```python
from build123d import *

# Parameters (mm, degrees)
F1_DEPTH = 10
F3_DEPTH = 4
F4_DEPTH = 4


with BuildPart() as f1:
    # F0 (on Top) → F1 (new body)
    with BuildSketch(Plane.XY):
        with BuildLine():
            Line((115, 150), (115, 0))
            Line((115, 0), (125, 0))
            Line((125, 0), (125, 150))
            ThreePointArc((125, 150), (0, 185), (-125, 150))
            Line((-125, 150), (-125, 0))
            Line((-125, 0), (-115, 0))
            Line((-115, 0), (-115, 150))
            Line((-115, 150), (-104.454365, 150))
            ThreePointArc((-104.454365, 150), (0, 175), (104.454365, 150))
            Line((104.454365, 150), (115, 150))
        make_face()
        with BuildLine():
            Line((-115, 0), (115, 0))
            Line((115, 0), (115, 150))
            Line((115, 150), (104.454365, 150))
            ThreePointArc((104.454365, 150), (0, 175), (-104.454365, 150))
            Line((-104.454365, 150), (-115, 150))
            Line((-115, 150), (-115, 0))
        make_face()
    extrude(amount=F1_DEPTH)

    # F2 (on face) → F3 (cut)
    with BuildSketch(Plane.XY.offset(10)):
        with BuildLine():
            Line((-115, 150), (-115, 0))
            Line((-115, 0), (115, 0))
            Line((115, 0), (115, 150))
            Line((115, 150), (104.454365, 150))
            ThreePointArc((104.454365, 150), (0, 175), (-104.454365, 150))
            Line((-104.454365, 150), (-115, 150))
        make_face()
    extrude(amount=-F3_DEPTH, mode=Mode.SUBTRACT)

    # F0 (on Top) → F4 (cut)
    with BuildSketch(Plane.XY):
        with BuildLine():
            Line((-115, 0), (115, 0))
            Line((115, 0), (115, 150))
            Line((115, 150), (104.454365, 150))
            ThreePointArc((104.454365, 150), (0, 175), (-104.454365, 150))
            Line((-104.454365, 150), (-115, 150))
            Line((-115, 150), (-115, 0))
        make_face()
    extrude(amount=F4_DEPTH, mode=Mode.SUBTRACT)


solid = f1.part
```
Verification items for the finished model (mm, model axes). A direction names the side the tool comes from. Give positions to 0.01 mm unless a question says otherwise; leave off trailing zeros. Order: outer loops, then holes, each group sorted by start corner. A loop starts at its lowest first (then second) coordinate and runs counter-clockwise, first axis right, second up. Notation, with made-up numbers: M 69,-36 L 99,-36 A21 cw 99,-5 Z; hole C 72.25,-4.5 d6. An arc over 180 degrees is marked long. Answer in a Markdown table with one row per item. Add a question column.
Item 1: Section check A-A, the plane y = 66. Enter the section's corners in (x, z), and give its area (3 significant figures).
Item 2: Gauge pin test, flat ends, axial feed: pin 1 (2 mm diameter, centred on x = 111.5, z = 9, fed in from -Y); pin 2 (6 mm diameter, centred on y = 164, z = 7, fed in from -X); pin 3 (2 mm diameter, centred on x = -92.5, y = 59, fed in from -Z); pin 4 (4.5 mm diameter, centred on x = 109, z = 2.5, fed in from -Y). Record the tip position at first contact, or that the pin passes through.
Item 3: Mould release check, pull along X, two halves, no side actions. Record for faces 1 (the flat face through (-0.6, 175.2, 0)), 2 (the cylindrical face through (1.84, 184.993, 4.93)), 3 (the cylindrical face through (1.518, 174.995, 1.972)): released by +X, released by -X, zero draft, split by the parting line, or undercut.
Item 4: Section check B-B, the plane x = 101.5. Enter the section's corners in (y, z), and give its area (3 significant figures).
Item 5: Scan lines: probe 1 along X at (y, z) = (145, 8.75); probe 2 along Z at (x, y) = (98, 54); probe 3 along X at (y, z) = (155, 2.5). Record each from-to range of solid material in increasing order. Write a range as from..to.
Item 6: Section check D-D, the plane y = 154.5. Enter the section's corners in (x, z).
Item 7: Section check C-C, the plane x = 55. Enter the section's corners in (y, z), and give its area (3 significant figures).
Item 8: Tool access check on faces 4 (the cylindrical face through (1.518, 174.995, 8.028)), 5 (the flat face through (-2, 89, 4)), 6 (the flat face through (-1, 0, 5)). Record the directions out of +Z, -Z, +X, -X, +Y, -Y that give a thin tool (end or side, any length) a straight path to the whole face; none if there is none.
Filled sheet:
| question | item | result |
|---|---|---|
| 1 | outline | M -125,0 L -115,0 L -115,4 L 115,4 L 115,0 L 125,0 L 125,10 L 115,10 L 115,6 L -115,6 L -115,10 L -125,10 Z |
| 1 | area | 660 mm^2 |
| 2 | pin 1 | stops at y = 150 |
| 2 | pin 2 | stops at x = -104.78 |
| 2 | pin 3 | stops at z = 4 |
| 2 | pin 4 | stops at y = 0 |
| 3 | face 1 | zero draft |
| 3 | face 2 | split by the parting line |
| 3 | face 3 | undercut |
| 4 | outline | M 0,4 L 151.47,4 L 151.47,0 L 162.55,0 L 162.55,10 L 151.47,10 L 151.47,6 L 0,6 Z |
| 4 | area | 414 mm^2 |
| 5 | probe 1 | x = -125..-115, 115..125 |
| 5 | probe 2 | z = 4..6 |
| 5 | probe 3 | x = -116.37..-93.96, 93.96..116.37 |
| 6 | outline | M -117.27,0 L -95.07,0 L -95.07,4 L 95.07,4 L 95.07,0 L 117.27,0 L 117.27,10 L 95.07,10 L 95.07,6 L -95.07,6 L -95.07,10 L -117.27,10 Z |
| 7 | outline | M 0,4 L 168.35,4 L 168.35,0 L 178.63,0 L 178.63,10 L 168.35,10 L 168.35,6 L 0,6 Z |
| 7 | area | 440 mm^2 |
| 8 | face 4 | +Z, -Y |
| 8 | face 5 | -Z, -Y |
| 8 | face 6 | +Z, -Z, +X, -X, -Y |
